Read the model definition and answer for the solid it produces. Units are mm, in the model's axes. A direction names the side the tool comes from. Give positions to 0.01 mm unless a question says otherwise; leave off trailing zeros. Order: outer loops, then holes, each group sorted by start corner. A loop starts at its lowest first (then second) coordinate and runs counter-clockwise, first axis right, second up. Notation, with made-up numbers: (3, 49.5) -> (22, 49.5) arc R10 cw to (22, 55.5) -> close; hole circle Ø6 at (-39.75, -36). An arc over 180 degrees is marked (long way). One line per question, with ' | ' between items. Start each with the question number.
```python
from build123d import *

# Parameters (mm, degrees)
SKETCH009_W             = 98.6
SKETCH009_H             = 84.6
PAD006_DEPTH            = 1.6
SKETCH010_W             = 98.6
SKETCH010_H             = 84.6
SKETCH010_W_2           = 96.6
SKETCH010_H_2           = 82.6
PAD007_DEPTH            = 6
SKETCH020_W             = 11.5
SKETCH020_H             = 15
PAD018_DEPTH            = 22.5
SKETCH027_W             = 3
SKETCH027_H             = 8
PAD019_DEPTH            = 17
SKETCH014_R             = 1.75
POCKET009_DEPTH         = 5
BODY003_PLACEMENT_ANGLE = 180


with BuildPart() as part:
    # Sketch009 → Pad006 (new body)
    with BuildSketch(Plane.XY):
        Rectangle(SKETCH009_W, SKETCH009_H)
    extrude(amount=PAD006_DEPTH)

    # Sketch010 → Pad007 (join)
    with BuildSketch(Plane.XY):
        Rectangle(SKETCH010_W, SKETCH010_H)
        Rectangle(SKETCH010_W_2, SKETCH010_H_2, mode=Mode.SUBTRACT)
    extrude(amount=PAD007_DEPTH)

    # Sketch020 → Pad018 (join)
    with BuildSketch(Plane.XY):
        with Locations((-40.95, 17.5)):
            Rectangle(SKETCH020_W, SKETCH020_H)
        with Locations((-40.95, -17.5)):
            Rectangle(SKETCH020_W, SKETCH020_H)
    extrude(amount=PAD018_DEPTH)

    # Sketch027 → Pad019 (join)
    with BuildSketch(Plane.XY):
        with Locations((45.2, 6)):
            Rectangle(SKETCH027_W, SKETCH027_H)
        with Locations((45.2, -6)):
            Rectangle(SKETCH027_W, SKETCH027_H)
    extrude(amount=PAD019_DEPTH)

    # Sketch014 → Pocket009 (cut)
    with BuildSketch(Plane.XY):
        with Locations((-44, 37)):
            Circle(SKETCH014_R)
        with Locations((12, 37)):
            Circle(SKETCH014_R)
        with Locations((44, 37)):
            Circle(SKETCH014_R)
        with Locations((44, -37)):
            Circle(SKETCH014_R)
        with Locations((12, -37)):
            Circle(SKETCH014_R)
        with Locations((-44, -37)):
            Circle(SKETCH014_R)
    extrude(amount=POCKET009_DEPTH, mode=Mode.SUBTRACT)


with BuildPart() as part_1:
    # Body003 placement: moved
    add(part.part.moved(Location((0, 0, 49.5))).rotate(Axis((0, 0, 49.5), (1, 0, 0)), BODY003_PLACEMENT_ANGLE))


solid = part_1.part
```
Q1. A cutting plane is placed at B-B, the plane y = -37. Determine the outline of the cut face in (x, z).
Q2. A cutting plane is placed at C-C, the plane x = -44. Determine the outline of the cut face in (y, z), then the cut area to 3 significant figures.
Q3. Find the intervals of material crossed by line 1 (X direction, y = -37, z = 48.95); line 2 (Y direction, x = 44, z = 48.7); line 3 (X direction, y = 33, z = 47.5), in increasing order.
Q4. Given P1, Ø6.5, axis at y = 5, z = 43, coming from the +X side; P2, Ø2.5, axis at x = 45, z = 36.5, coming from the -Y side; P3, Ø8, axis at y = -12.5, z = 36, coming from the +X side; P4, Ø5, axis at x = 33, y = -3, coming from the -Z side, each flat-ended and moving along its own axis, determine where each tip first touches the part or whether it passes through.
Q5. Which of the six approach directions +Z, -Z, +X, -X, +Y, -Y give full straight-line access (tool end or side, diameter ignored) to faces 4 (the flat face through (-46.7, 18, 38)), 5 (the cylindrical face through (-42.383, 37.67, 48.711))?
Q6. A cutting plane is placed at D-D, the plane y = 21. Determine the outline of the cut face in (x, z), then the cut area to 3 significant figures.
Q7. Determine the mould class of faces 1 (the flat face through (-41, -18, 27)), 2 (the flat face through (49.3, 1, 47)), 3 (the flat face through (-35.2, 18, 38)) for opening direction X: pulls with the +X half, pulls with the -X half, needs draft (parallel to the pull), parting line crosses it, or undercut.
Q8. A cutting plane is placed at A-A, the plane z = 45.25. Determine the outline of the cut face in (x, y), then the cut area to 3 significant figures.
Geometry results:
1) outline: (-49.3, 43.5) -> (-48.3, 43.5) -> (-48.3, 47.9) -> (-45.75, 47.9) -> (-45.75, 49.5) -> (-49.3, 49.5) -> close; (-42.25, 47.9) -> (10.25, 47.9) -> (10.25, 49.5) -> (-42.25, 49.5) -> close; (13.75, 47.9) -> (42.25, 47.9) -> (42.25, 49.5) -> (13.75, 49.5) -> close; (45.75, 47.9) -> (48.3, 47.9) -> (48.3, 43.5) -> (49.3, 43.5) -> (49.3, 49.5) -> (45.75, 49.5) -> close
2) outline: (-42.3, 43.5) -> (-41.3, 43.5) -> (-41.3, 47.9) -> (-38.75, 47.9) -> (-38.75, 49.5) -> (-42.3, 49.5) -> close; (-35.25, 47.9) -> (-25, 47.9) -> (-25, 27) -> (-10, 27) -> (-10, 47.9) -> (10, 47.9) -> (10, 27) -> (25, 27) -> (25, 47.9) -> (35.25, 47.9) -> (35.25, 49.5) -> (-35.25, 49.5) -> close; (38.75, 47.9) -> (41.3, 47.9) -> (41.3, 43.5) -> (42.3, 43.5) -> (42.3, 49.5) -> (38.75, 49.5) -> close | area: 760 mm²
3) line 1: -49.3 to -45.75, -42.25 to 10.25, 13.75 to 42.25, 45.75 to 49.3 | line 2: -42.3 to -38.75, -35.25 to 35.25, 38.75 to 42.3 | line 3: -49.3 to -48.3, 48.3 to 49.3
4) P1: x = 49.3 | P2: y = -10 | P3: x = 46.7 | P4: z = 47.9
5) face 4: -Z | face 5: +Z, -Z
6) outline: (-49.3, 43.5) -> (-48.3, 43.5) -> (-48.3, 47.9) -> (-46.7, 47.9) -> (-46.7, 27) -> (-35.2, 27) -> (-35.2, 47.9) -> (48.3, 47.9) -> (48.3, 43.5) -> (49.3, 43.5) -> (49.3, 49.5) -> (-49.3, 49.5) -> close | area: 407 mm²
7) face 1: needs draft | face 2: pulls with the +X half | face 3: undercut
8) outline: (-49.3, -42.3) -> (49.3, -42.3) -> (49.3, 42.3) -> (-49.3, 42.3) -> close; (-46.7, -25) -> (-35.2, -25) -> (-35.2, -10) -> (-46.7, -10) -> close; (-46.7, 10) -> (-35.2, 10) -> (-35.2, 25) -> (-46.7, 25) -> close; (43.7, -10) -> (46.7, -10) -> (46.7, -2) -> (43.7, -2) -> close; (43.7, 2) -> (46.7, 2) -> (46.7, 10) -> (43.7, 10) -> close; hole (-48.3, -41.3) -> (48.3, -41.3) -> (48.3, 41.3) -> (-48.3, 41.3) -> close | area: 755 mm²
